Read the model definition and answer for the solid it produces. Units are mm, in the model's axes. A direction names the side the tool comes from. Give positions to 0.01 mm unless a question says otherwise; leave off trailing zeros. Loops run counter-clockwise (first coordinate to the right, second up) from the corner with the lowest first, then second, coordinate; pieces in that order, holes last. Notation, with made-up numbers: (87, -22.75) - (128, -22.75) arc R5 cw to (128, -18.75) - close; hole circle Ø7 at (45, -18). An arc over 180 degrees is marked (long way). Write each question's results on one line, items separated by ' | '. Start each with the question number.
Q1. For faces 1 (the flat face through (0, 9.525, 282)), 2 (the cylindrical face through (-0.731, -11.09, 335.182)), determine the directions among +Z, -Z, +X, -X, +Y, -Y from which every point of the face is accessible in a straight line to the end or side of a thin tool.
Q2. The part is cut by section A-A, the plane z = 363.5. Write down the section's boundary in (x, y) (3 decimals).
Q3. Find the intervals of material crossed by line 1 (X direction, y = 2.5, z = 400.5) (3 decimals); line 2 (Y direction, x = 11.05, z = 165.75), in increasing order. Write a range as from..to.
Q4. Determine the mould class of faces 3 (the flat face through (11, 0, 571.5)), 4 (the cylindrical face through (-0.731, 11.135, 262.157)), 5 (the flat face through (-12.7, 0, 282)) for opening direction X: +X half, -X half, draft (parallel to the pull), parting line (faces both ways), or undercut.
Q5. Given pin 1 (4 mm diameter, centred on x = 0, z = 514.35, fed in from +Y), flat-ended and moving along its own axis, determine where the tip first touches the part or whether it passes through.
```python
from build123d import *

# Parameters (mm, degrees)
SKETCH1_W                    = 25.4
SKETCH1_H                    = 25.4
SKETCH1_W_2                  = 19.05
SKETCH1_H_2                  = 19.05
EXTRUDE_THIN1_DEPTH          = 571.5
F_8_CLEARANCE_HOLE1_D        = 4.4958
F_8_32_TAPPED_HOLE1_D        = 3.4544
F_8_32_TAPPED_HOLE1_DEPTH    = 10.70864
F_8_32_TAPPED_HOLE1_TIP      = 1.037806461
F_3_8_0_375_DIAMETER_HOLE2_D = 9.525


with BuildPart() as part:
    # Sketch1 → Extrude-Thin1 (new body)
    with BuildSketch(Plane.XY):
        Rectangle(SKETCH1_W, SKETCH1_H)
        Rectangle(SKETCH1_W_2, SKETCH1_H_2, mode=Mode.SUBTRACT)
    extrude(amount=EXTRUDE_THIN1_DEPTH)

    # #8 Clearance Hole1 (through all)
    with Locations(Plane(origin=(0, 12.7, 565.15), x_dir=(0, 0, 1), z_dir=(0, 1, 0))):
        with Locations((0, 0), (-558.8, 0), (-533.4, 0), (-508, 0), (-25.4, 0), (-50.8, 0)):
            Hole(F_8_CLEARANCE_HOLE1_D / 2)

    # #8-32 Tapped Hole1
    with Locations(Plane(origin=(12.7, 82.55, 285.75), x_dir=(0, 0, 1), z_dir=(1, 0, 0))):
        with Locations((-300, 82.55), (-240, 82.55), (-180, 82.55), (-60, 82.55), (0, 82.55), (60, 82.55), (120, 82.55), (180, 82.55), (240, 82.55), (-120, 82.55), (-360, 82.55), (300, 82.55), (360, 82.55)):
            Hole(F_8_32_TAPPED_HOLE1_D / 2, depth=F_8_32_TAPPED_HOLE1_DEPTH)
            with Locations((0, 0, -(F_8_32_TAPPED_HOLE1_DEPTH + F_8_32_TAPPED_HOLE1_TIP / 2))):  # 118° drill point
                Cone(0, F_8_32_TAPPED_HOLE1_D / 2, F_8_32_TAPPED_HOLE1_TIP, mode=Mode.SUBTRACT)

    # 3/8 (0.375) Diameter Hole2 (through all)
    with Locations(Plane(origin=(-346.075, -12.7, 285.75), x_dir=(0, 0, 1), z_dir=(0, -1, 0))):
        with Locations((-92.583, 346.075), (-35.433, 346.075), (35.814, 346.075), (92.964, 346.075), (-19.05, -346.775), (53.975, -346.775), (127, -346.775), (-381, -114.3), (-381, -130.175), (-381, -146.05), (-381, 114.3), (-381, 98.425), (-381, 82.55)):
            Hole(F_3_8_0_375_DIAMETER_HOLE2_D / 2)


solid = part.part
```
Check sheet entries:
1) face 1: +Z, -Z | face 2: +Y, -Y
2) outline: (-12.7, -12.7) - (12.7, -12.7) - (12.7, 12.7) - (-12.7, 12.7) - close; hole (-9.525, -9.525) - (9.525, -9.525) - (9.525, 9.525) - (-9.525, 9.525) - close
3) line 1: x = -12.7..-9.525, 9.525..12.7 | line 2: y = -12.7..-1.73, 1.73..12.7
4) face 3: draft | face 4: undercut | face 5: -X half
5) pin 1: passes through
